Answer from the drawing. Dimensions are ordinates in mm from the lowest x, y and z of the part. Give positions to 0.01 mm unless a question says otherwise; leave off trailing zeros. Loops run counter-clockwise (first coordinate to the right, second up) from the corner with the lowest first, then second, coordinate; pieces in that order, holes last.
Item 1: Each of these flat-tipped pins is pushed along its axis until it touches: pin 1 Ø1 at (y, z) = (1, 20) entering from -X; pin 2 Ø0.5 at (x, y) = (16, 1) entering from -Z. Where does it stop, or does it pass through?
Item 2: Section B-B, the plane z = 7 is taken. Give the vertices of the cut face in (x, y) (1 decimal), and give its area (3 significant figures).
Item 3: Consider line 1 along X through (y, z) = (0.8, 11.5) (1 decimal); line 2 along Z through (x, y) = (3.5, 0.8); line 3 along Z through (x, y) = (13.5, 1.85) (1 decimal). Determine where each line is inside the solid, lowest interval first.
Item 4: Section A-A, the plane y = 1.3 is taken. Give the vertices of the cut face in (x, z) (1 decimal).
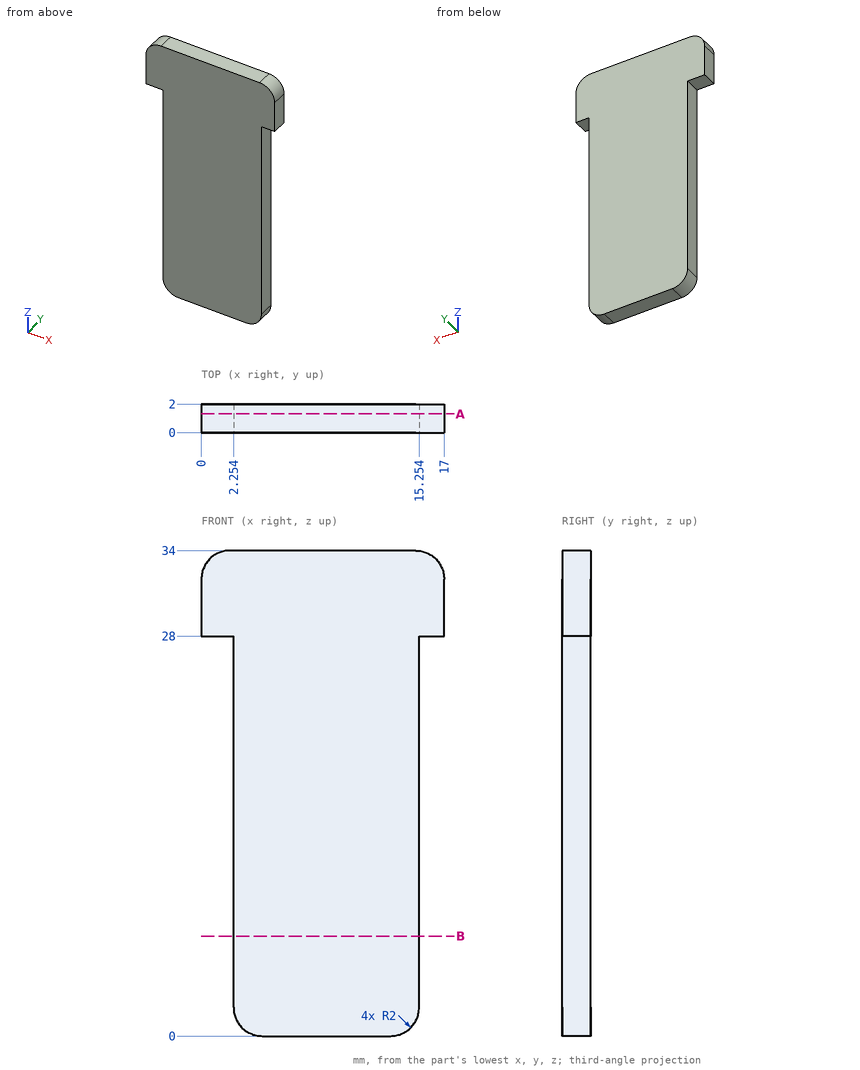
Worked answers:
1. pin 1: stops at x = 2.25
1. pin 2: stops at z = 28
2. outline: (2.3, 0) - (15.3, 0) - (15.3, 2) - (2.3, 2) - close
2. area: 26.0 mm2
3. line 1: x = 2.3 to 15.3
3. line 2: z = 0.15 to 34
3. line 3: z = 0 to 34
4. outline: (0, 28) - (2.3, 28) - (2.3, 2) arc R2 ccw to (4.3, 0) - (13.3, 0) arc R2 ccw to (15.3, 2) - (15.3, 28) - (17, 28) - (17, 32) arc R2 ccw to (15, 34) - (2, 34) arc R2 ccw to (0, 32) - close
